The listing builds one solid part. Answer for the finished solid, in the listing's coordinates (mm). A direction names the side the tool comes from. Coordinates: 2 decimals unless noted, no trailing zeros. Loops run counter-clockwise (first coordinate to the right, second up) from the corner with the lowest first, then second, coordinate; pieces in that order, holes last. Notation, with made-up numbers: M 25,5.25 L 67,5.25 A20 cw 67,33.25 Z; hole C -18,15.25 d8. An arc over 180 degrees is marked long. Answer as CSV lines item,"result". Start each with the question number.
Autodesk Inventor part; units mm, degrees
ref_plane "YZ Plane" through (0, 0, 0) normal (1, 0, 0) x (0, 1, 0)
ref_plane "XZ Plane" through (0, 0, 0) normal (0, 1, 0) x (-1, 0, 0)
ref_plane "XY Plane" through (0, 0, 0) normal (0, 0, 1) x (1, 0, 0)
sketch "Sketch2" plane through (0, 0, 0) normal (0, 0, 1) x (1, 0, 0)
  line L0 (-40, 16) -> (40, 16)
  line L1 (40, 16) -> (40, -16)
  line L2 (40, -16) -> (-40, -16)
  line L3 (-40, -16) -> (-40, 16)
  line L4 (-40, 16) -> (40, -16) construction
  line L5 (40, 16) -> (-40, -16) construction
  point P0 (0, 0)
  dimension "d4" = 32
  dimension "d5" = 80
extrude "Extrusion1" add sketch "Sketch2" along normal blind 26
sketch "Sketch6" plane through (-40, 16, 0) normal (0, 1, 0) x (1, 0, 0)
  line L0 (12, -9.5) -> (0, -9.5) construction
  line L1 (0, 0) -> (0, -26)
  line L2 (68, -9.5) -> (80, -9.5) construction
  line L3 (80, 0) -> (80, -26)
  line L4 (80, 0) -> (0, 0)
  point P0 (40, 0)
  point P1 (74, -9.5)
  dimension "d29" = 56
  dimension "d30" = 9.5
hole "Hole3" at (-28, 16, 9.5) at (28, 16, 9.5) direction (0, -1, 0) diameter 8.2 end through all
sketch "Sketch9" plane through (-40, 16, 0) normal (0, 1, 0) x (1, 0, 0)
  line L0 (0, 0) -> (0, -26)
  line L1 (80, -26) -> (0, -26)
  line L2 (0, 0) -> (80, -26)
  point P0 (40, 0)
sketch "Sketch10" plane through (-40, 16, 0) normal (0, 1, 0) x (1, 0, 0)
  point P0 (40, 0)
sketch "Sketch11" plane through (40, -16, 0) normal (1, 0, 0) x (0, 0, -1)
  line L0 (0, 0) -> (0, 32)
  line L1 (0, 0) -> (-26, 0)
  line L2 (-26, 0) -> (-26, 200)
  line L3 (-26, 200) -> (0, 200)
  line L4 (0, 200) -> (0, 0)
  line L5 (-26, 0) -> (-26, 32)
  point P0 (0, 16)
  dimension "d52" = 200
extrude "Extrusion4" add sketch "Sketch11" along normal blind 32
fillet "Fillet1" radius 10 1 edges at (72, -16, 13)
sketch "Sketch13" plane through (40, 184, 26) normal (0, 1, 0) x (1, 0, 0)
  line L0 (32, 26) -> (-30, 26)
  line L1 (0, 26) -> (-80, 26)
  line L2 (32, 26) -> (32, 0)
  line L3 (32, 26) -> (32, -36)
  line L4 (-30, 26) -> (32, -36)
  point P0 (-40, 26)
  dimension "d58" = 62
extrude "Extrusion5" add sketch "Sketch13" against normal blind 10
fillet "Fillet2" radius 5 1 edges at (10, 179, 0)
fillet "Fillet3" radius 5 1 edges at (72, 179, 62)
sketch "Sketch15" plane through (22.0711, 184, 0) normal (0, 1, 0) x (1, 0, 0)
  line L0 (0, 0) -> (49.9289, 0)
  line L1 (49.9289, 0) -> (49.9289, -26)
  line L2 (49.9289, 0) -> (17.9289, 0)
  line L3 (17.9289, 0) -> (17.9289, -32)
  line L4 (17.9289, -32) -> (49.9289, -32)
  line L5 (49.9289, -32) -> (49.9289, 0)
  line L6 (49.9289, 0) -> (49.9289, -49.9289)
  point P0 (-22.0711, 0)
  point P1 (41.9289, -42)
  point P2 (7.9289, -8)
  dimension "d63" = 8
  dimension "d64" = 32
  dimension "d65" = 32
  dimension "d66" = 10
  dimension "d67" = 10
  dimension "d68" = 8
hole "Hole6" at (30, 184, 8) at (64, 184, 42) direction (0, -1, 0) diameter 8.2 depth 20
properties part number "13042026-12"
Item 1: Section B-B on z = 42 is taken. Determine the outline of the cut face in (x, y), then the cut area to 3 significant figures.
Item 2: Section D-D on x = 53 is taken. Determine the outline of the cut face in (y, z).
Item 3: Section C-C on z = 18.5 is taken. Determine the outline of the cut face in (x, y), then the cut area to 3 significant figures.
Item 4: Section A-A on x = 37.5 is taken. Determine the outline of the cut face in (y, z).
Item 5: Consider line 1 (Z direction, x = -28, y = -2.5); line 2 (X direction, y = 13.5, z = 8.5); line 3 (Y direction, x = 4.5, z = 15). Determine where each line is inside the solid, lowest interval first.
Item 6: Each of these flat-tipped pins is pushed along its axis until it touches: P1, Ø2, axis at y = 32, z = 24, coming from the -X side; P2, Ø6.5, axis at x = 28, z = 9.5, coming from the -Y side; P3, Ø7.5, axis at x = 64, z = 42, coming from the +Y side; P4, Ø21, axis at x = -12, z = 12, coming from the +Y side. Where does it stop, or does it pass through?
Item 7: For faces 1 (the face through (53, 57, 26)), 2 (the face through (17.42, 178.93, 3.16)), 3 (the face through (40, 96, 13)), 4 (the face through (44, 174, 27)), determine the directions among +Z, -Z, +X, -X, +Y, -Y from which every point of the face is accessible in a straight line to the end or side of a thin tool.
Item 8: For a pull along Z with two mould halves and no side action, classify faces 5 (the face through (-24, -0.2, 8.6)), 6 (the face through (68.989, 178.93, 54.516)), 7 (the face through (50, 184, 22)) as pulls with the +Z half, pulls with the -Z half, needs draft (parallel to the pull), parting line crosses it, or undercut.
Results are:
1,outline,"M 52,174 L 59.9,174 L 59.9,184 L 52,184 Z; M 68.1,174 L 72,174 L 72,184 L 68.1,184 Z"
1,area,"118 mm²"
2,outline,"M -16,0 L 184,0 L 184,43 L 174,43 L 174,26 L -16,26 Z"
3,outline,"M -40,-16 L 62,-16 A10 ccw 72,-6 L 72,184 L 28.5,184 L 28.5,174 L 40,174 L 40,16 L -40,16 Z"
3,area,"9,050 mm²"
4,outline,"M -16,0 L 16,0 L 16,26 L -16,26 Z; M 174,0 L 184,0 L 184,27.5 L 174,27.5 Z"
5,line 1,"0 to 5.4, 13.6 to 26"
5,line 2,"-40 to -31.98, -24.02 to 24.02, 31.98 to 72"
5,line 3,"-16 to 16"
6,P1,"x = 40"
6,P2,"y = 174"
6,P3,"through"
6,P4,"y = 16"
7,face 1,"+Z, +X, -X, -Y"
7,face 2,"-X, +Y"
7,face 3,"+Z, -Z, -X"
7,face 4,"+Z, -X"
8,face 5,"undercut"
8,face 6,"pulls with the +Z half"
8,face 7,"needs draft"
